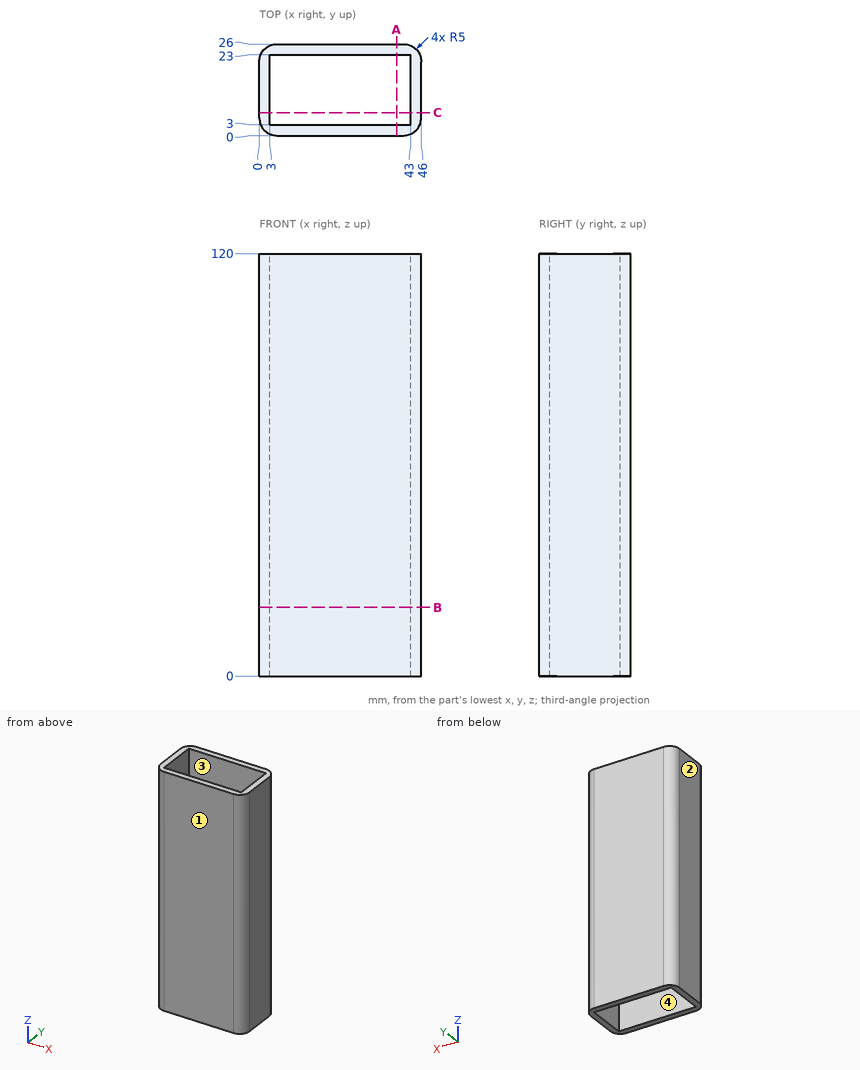
Study the drawing (mm; zero at the part's minimum x, y, z) and answer. Give positions to 0.01 mm unless a question says otherwise; leave off trailing zeros. Order: outer loops, then holes, each group sorted by start corner. A loop starts at its lowest first (then second) coordinate and runs counter-clockwise, first axis right, second up. Notation, with made-up numbers: (-5.75, 11) - (48.25, 11) arc R25 cw to (48.25, 40) - close; hole circle Ø11 at (-37.5, -12). An arc over 180 degrees is marked (long way). Answer as CSV lines item,"result". Start each with the question number.
Q1. The part is cut by section A-A (x = 39). Write down the section's boundary in (y, z), then the cut area to 3 significant figures.
Q2. The part is cut by section B-B (z = 19.5). Write down the section's boundary in (x, y), then the cut area to 3 significant figures.
Q3. Given pin 1 Ø12 at (x, y) = (33, 16.5) entering from +Z, flat-ended and moving along its own axis, determine where the tip first touches the part or whether it passes through.
Q4. Find the intervals of material crossed by L1, parallel to Y at x = 15.5, z = 48; L2, parallel to X at y = 5, z = 44.5; L3, parallel to X at y = 22.75, z = 12.5, in increasing order. Write a range as [from, to].
Q5. The part is cut by section C-C (y = 6.5). Write down the section's boundary in (x, z).
Q6. The mould has two halves that part along X. Classify the marked faces 1, 2, 3 and 4: +X half, -X half, draft (parallel to the pull), parting line (faces both ways), or undercut.
Check result:
1,outline,"(0, 0) - (3, 0) - (3, 120) - (0, 120) - close; (23, 0) - (26, 0) - (26, 120) - (23, 120) - close"
1,area,"720 mm²"
2,outline,"(0, 5) arc R5 ccw to (5, 0) - (41, 0) arc R5 ccw to (46, 5) - (46, 21) arc R5 ccw to (41, 26) - (5, 26) arc R5 ccw to (0, 21) - close; hole (3, 3) - (43, 3) - (43, 23) - (3, 23) - close"
2,area,"375 mm²"
3,pin 1,"passes through"
4,L1,"y = [0, 3], [23, 26]"
4,L2,"x = [0, 3], [43, 46]"
4,L3,"x = [0.32, 3], [43, 45.68]"
5,outline,"(0, 0) - (3, 0) - (3, 120) - (0, 120) - close; (43, 0) - (46, 0) - (46, 120) - (43, 120) - close"
6,face 1,"draft"
6,face 2,"-X half"
6,face 3,"undercut"
6,face 4,"undercut"
